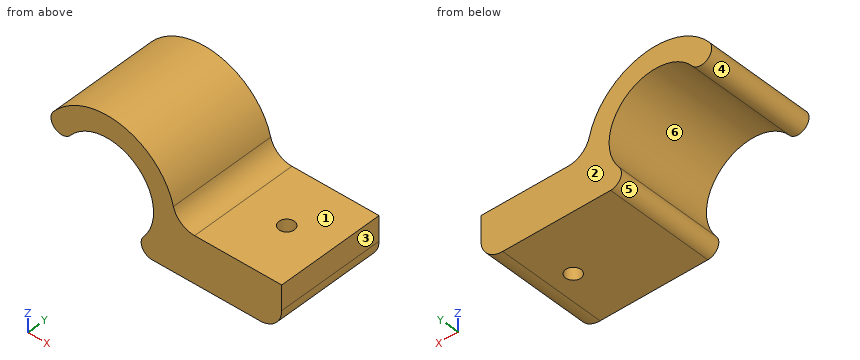
```python
from build123d import *

# Parameters (mm, degrees)
F1_DEPTH = 12.5
F2_R     = 5
F3_R     = 1.75
F4_DEPTH = 10.669


with BuildPart() as f1:
    # F0 (on Front) → F1 (new body, symmetric)
    with BuildSketch(Plane.XZ):
        with BuildLine():
            ThreePointArc((-8.367673, 6.617271), (6.617271, 8.367673), (8.367673, -6.617271))
            ThreePointArc((8.367673, -6.617271), (8.078399, -9.257307), (10.328601, -10.668))
            Line((10.328601, -10.668), (40, -10.668))
            Line((40, -10.668), (40, 0))
            Line((40, 0), (15.668, 0))
            ThreePointArc((15.668, 0), (5.144603, 14.7993), (-12.289529, 9.718729))
            ThreePointArc((-12.289529, 9.718729), (-11.87933, 6.207072), (-8.367673, 6.617271))
        make_face()
    extrude(amount=F1_DEPTH, both=True)

    # F2
    f2_edges = [f1.edges().sort_by_distance(p)[0] for p in [
        (15.668, 0, 0),
        (40, 0, -10.668),
    ]]
    fillet(f2_edges, radius=F2_R)

    # F3 (on Top) → F4 (cut, through all)
    with BuildSketch(Plane.XY):
        with Locations((30, 0)):
            Circle(F3_R)
    extrude(amount=-F4_DEPTH, mode=Mode.SUBTRACT)


solid = f1.part
```
For this review, take the finished solid that the model builds, in its own axes (mm). Face numbers are marked on the shaded views. A direction names the side the tool comes from. Round coordinates to 2 decimals unless told otherwise and drop trailing zeros. Write each loop counter-clockwise with the first axis right and the second up, starting at its lowest first coordinate (ties: lowest second). Pieces come first, ordered by that corner, then holes. Notation, with made-up numbers: (32, 38.25) - (82, 38.25) arc R21 cw to (82, 73.25) - close; hole circle Ø1 at (29.5, 78.25). An arc over 180 degrees is marked (long way). Put each result on its own line as item: value.
Q1. Machinability: for the marked faces 1 and 2, which of the approach directions +Z, -Z, +X, -X, +Y, -Y give a long, thin tool a straight path to every point of the face, cutting with its end or side? Answer none if there is none.
Solved:
face 1: +Z, +X, +Y, -Y
face 2: +Z, -Z, +X, -X, +Y
Q2. We need section A-A (x = 30). Give the boundary of the cut face in (y, z).
Solved:
outline: (-12.5, -10.67) - (-1.75, -10.67) - (-1.75, 0) - (-12.5, 0) - close; (1.75, -10.67) - (12.5, -10.67) - (12.5, 0) - (1.75, 0) - close
Q3. Mouldability with a two-part tool opening along X and no side actions: class the marked faces 3, 4, 5 and 6 as released by +X, released by -X, zero draft, split by the parting line, or undercut.
Solved:
face 3: released by +X
face 4: undercut
face 5: released by -X
face 6: undercut
Q4. Insertion check: pin 1 Ø1.5 at (y, z) = (-4, -8) entering from +X; pin 2 Ø5 at (y, z) = (6, 0) entering from -X; pin 3 Ø10 at (x, y) = (29, -0.5) entering from +Z; pin 4 Ø2 at (x, y) = (-1, 9.5) entering from +Z. Each pin has a flat end and moves straight along its axis. Give the tip position at first contact, or say it passes through.
Solved:
pin 1: stops at x = 39.74
pin 2: stops at x = 10.37
pin 3: stops at z = 0
pin 4: stops at z = 15.67
Q5. We need section B-B (y = 0). Give the boundary of the cut face in (x, z), and give its area (3 significant figures).
Solved:
outline: (-12.29, 9.72) arc R2.5 ccw to (-8.37, 6.62) arc R10.67 cw to (8.37, -6.62) arc R2.5 ccw to (10.33, -10.67) - (28.25, -10.67) - (28.25, 0) - (20.05, 0) arc R5 cw to (15.2, 3.79) arc R15.67 ccw to start; (31.75, -10.67) - (35, -10.67) arc R5 ccw to (40, -5.67) - (40, 0) - (31.75, 0) - close
area: 461 mm2
Q6. We need section D-D (y = -8.25). Give the boundary of the cut face in (x, z).
Solved:
outline: (-12.29, 9.72) arc R2.5 ccw to (-8.37, 6.62) arc R10.67 cw to (8.37, -6.62) arc R2.5 ccw to (10.33, -10.67) - (35, -10.67) arc R5 ccw to (40, -5.67) - (40, 0) - (20.05, 0) arc R5 cw to (15.2, 3.79) arc R15.67 ccw to start
Q7. We need section C-C (x = 0). Give the boundary of the cut face in (y, z), and give its area (3 significant figures).
Solved:
outline: (-12.5, 10.67) - (12.5, 10.67) - (12.5, 15.67) - (-12.5, 15.67) - close
area: 125 mm2
Q8. Wall thickness on probe 1 along Y at (x, z) = (30, -8); probe 2 along X at (y, z) = (-5.75, 7.75); probe 3 along Z at (x, y) = (20, -9): over which ranges is each line inside the solid? List them lowest first.
Solved:
probe 1: y = -12.5 to -1.75, 1.75 to 12.5
probe 2: x = -12.79 to -7.33, 7.33 to 13.62
probe 3: z = -10.67 to 0
